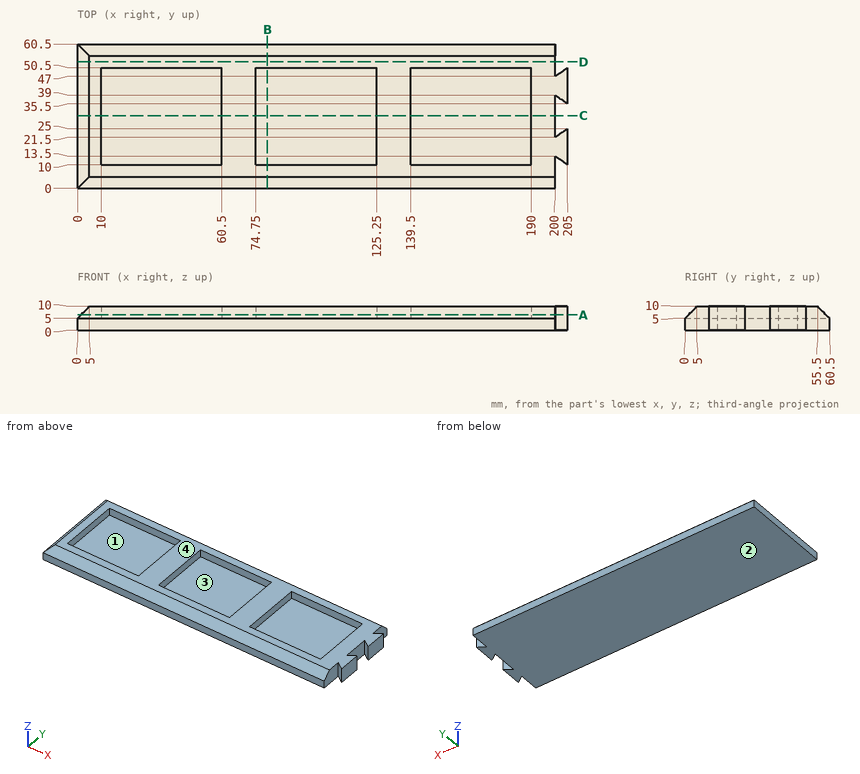
The drawing under review shows one solid part. Ordinate dimensions are in mm from its lowest x, y, z. A direction names the side the tool comes from. Coordinates: 2 decimals unless noted, no trailing zeros. Write each loop counter-clockwise with the first axis right and the second up, starting at its lowest first coordinate (ties: lowest second). Pieces come first, ordered by that corner, then holes. Notation, with made-up numbers: (9.5, 19.5) - (56.5, 19.5) arc R23 cw to (56.5, 27.5) - close; hole circle Ø10 at (83.25, 24). An arc over 180 degrees is marked (long way). Answer in a Markdown table with one row per item. Add a question column.
Q1. We need section A-A, the plane z = 6.5. State the section outline as (x, y) points.
Q2. For probe 1 along X at (y, z) = (14, 9.5); probe 2 along X at (y, z) = (19.5, 8.25); probe 3 along X at (y, z) = (3, 1.25), list the stretches that pass through material, from the lowest coordinate up.
Q3. Draft analysis for pull direction X (two halves, no side actions). For the marked faces 3 and 4, state which applies: +X half, -X half, draft (parallel to the pull), parting line (faces both ways), or undercut.
Q4. We need section D-D, the plane y = 53. State the section outline as (x, z) points, and give its area (3 significant figures).
Q5. We need section C-C, the plane y = 30.5. State the section outline as (x, z) points, and give its area (3 significant figures).
Q6. For P1, Ø5, axis at x = 125, z = 8.5, coming from the +Y side; P2, Ø1.5, axis at x = 26.5, z = 7, coming from the -Y side; P3, Ø2.5, axis at x = 104.5, z = 7.5, coming from the +Y side, all flat-tipped, find the tip position at first contact; note any pin that passes through.
Q7. We need section B-B, the plane x = 79.5. State the section outline as (y, z) points, and give its area (4 significant figures).
Q8. Tool access review of the marked faces 1 and 2: name each direction out of +Z, -Z, +X, -X, +Y, -Y from which nothing blocks a thin tool from reaching the whole face with its end or side.
Answer list:
| question | item | result |
|---|---|---|
| 1 | outline | (1.5, 1.5) - (200, 1.5) - (200, 13.5) - (205, 10) - (205, 25) - (200, 21.5) - (200, 39) - (205, 35.5) - (205, 50.5) - (200, 47) - (200, 59) - (1.5, 59) - close; hole (10, 10) - (60.5, 10) - (60.5, 50.5) - (10, 50.5) - close; hole (74.75, 10) - (125.25, 10) - (125.25, 50.5) - (74.75, 50.5) - close; hole (139.5, 10) - (190, 10) - (190, 50.5) - (139.5, 50.5) - close |
| 2 | probe 1 | x = 4.5 to 10, 60.5 to 74.75, 125.25 to 139.5, 190 to 205 |
| 2 | probe 2 | x = 3.25 to 10, 60.5 to 74.75, 125.25 to 139.5, 190 to 205 |
| 2 | probe 3 | x = 0 to 200 |
| 3 | face 3 | undercut |
| 3 | face 4 | draft |
| 4 | outline | (0, 0) - (200, 0) - (200, 10) - (5, 10) - (0, 5) - close |
| 4 | area | 1,990 mm2 |
| 5 | outline | (0, 0) - (200, 0) - (200, 10) - (190, 10) - (190, 5) - (139.5, 5) - (139.5, 10) - (125.25, 10) - (125.25, 5) - (74.75, 5) - (74.75, 10) - (60.5, 10) - (60.5, 5) - (10, 5) - (10, 10) - (5, 10) - (0, 5) - close |
| 5 | area | 1,230 mm2 |
| 6 | P1 | stops at y = 59.5 |
| 6 | P2 | stops at y = 1.25 |
| 6 | P3 | stops at y = 59.25 |
| 7 | outline | (0, 0) - (60.5, 0) - (60.5, 5) - (55.5, 10) - (50.5, 10) - (50.5, 5) - (10, 5) - (10, 10) - (5, 10) - (0, 5) - close |
| 7 | area | 377.5 mm2 |
| 8 | face 1 | +Z |
| 8 | face 2 | -Z, +X, -X, +Y, -Y |
